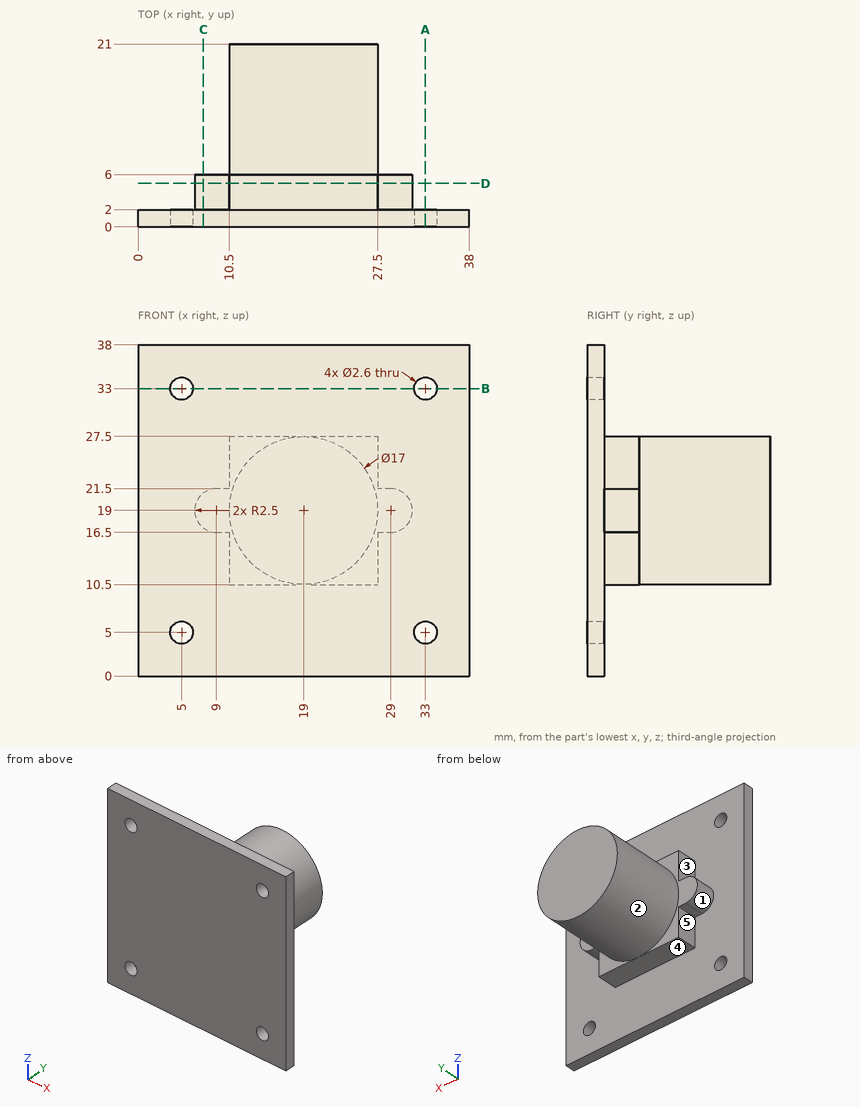
Design review of the part shown in the three views and the two pictorial views. Dimensions are in mm from the part's minimum x, y and z. A direction names the side the tool comes from. Give positions to 0.01 mm unless a question says otherwise; leave off trailing zeros. Write each loop counter-clockwise with the first axis right and the second up, starting at its lowest first coordinate (ties: lowest second). Pieces come first, ordered by that corner, then holes. Notation, with made-up numbers: M -25,80 L 6,80 A10 cw 6,97 Z; hole C -3.5,58.25 d3. An arc over 180 degrees is marked long. One line per item, written item: value.
1) Take a section at C-C, the plane x = 7.5. Write out the cut boundary in (y, z).
Results are:
outline: M 0,0 L 2,0 L 2,17 L 6,17 L 6,21 L 2,21 L 2,38 L 0,38 Z
2) Take a section at B-B, the plane z = 33. Write out the cut boundary in (x, y), then the cut area to 3 significant figures.
Results are:
outline: M 0,0 L 3.7,0 L 3.7,2 L 0,2 Z; M 6.3,0 L 31.7,0 L 31.7,2 L 6.3,2 Z; M 34.3,0 L 38,0 L 38,2 L 34.3,2 Z
area: 65.6 mm²
3) Take a section at A-A, the plane x = 33. Write out the cut boundary in (y, z), then the cut area to 3 significant figures.
Results are:
outline: M 0,0 L 2,0 L 2,3.7 L 0,3.7 Z; M 0,6.3 L 2,6.3 L 2,31.7 L 0,31.7 Z; M 0,34.3 L 2,34.3 L 2,38 L 0,38 Z
area: 65.6 mm²
4) For the marked faces 1, 2, 3, 4 and 5, list the 3-axis set-ups (+Z, -Z, +X, -X, +Y, -Y) from which the entire face can be reached by the end or side of a thin tool; tool diameter is ignored.
Results are:
face 1: -X, +Y
face 2: +Y
face 3: +Z, -X, +Y
face 4: -Z, +X, -X, +Y
face 5: -Z, -X, +Y
5) Take a section at D-D, the plane y = 5. Write out the cut boundary in (x, z), then the cut area to 3 significant figures.
Results are:
outline: M 9,16.5 L 10.5,16.5 L 10.5,10.5 L 27.5,10.5 L 27.5,16.5 L 29,16.5 A2.5 ccw 29,21.5 L 27.5,21.5 L 27.5,27.5 L 10.5,27.5 L 10.5,21.5 L 9,21.5 A2.5 ccw Z
area: 324 mm²
6) For P1, Ø0.8, axis at x = 9.5, y = 3, coming from the +Z side; P2, Ø1.2, axis at x = 28, y = 4.5, coming from the -Z side; P3, Ø2, axis at x = 33, z = 33, coming from the +Y side; P4, Ø4.5, axis at y = 4.5, z = 24.5, coming from the -X side, all flat-tipped, find the tip position at first contact; note any pin that passes through.
Results are:
P1: stops at z = 21.5
P2: stops at z = 10.5
P3: passes through
P4: stops at x = 10.5
7) For line 1 (Z direction, x = 33, y = 0.5); line 2 (Z direction, x = 11, y = 3.5), list the stretches that pass through material, from the lowest coordinate up. Write a range as from..to.
Results are:
line 1: z = 0..3.7, 6.3..31.7, 34.3..38
line 2: z = 10.5..27.5
